Build history of the part. All positions in model axes, mm. Face numbers are marked on the shaded views. A direction names the side the tool comes from. Round coordinates to 2 decimals unless told otherwise and drop trailing zeros. Write each loop counter-clockwise with the first axis right and the second up, starting at its lowest first coordinate (ties: lowest second). Pieces come first, ordered by that corner, then holes. Notation, with made-up numbers: (53, 56) - (90, 56) arc R33 cw to (90, 86) - close; hole circle Ø8 at (70, 72.25). An arc over 180 degrees is marked (long way). Answer as a JSON object with one key per item and string values. Group by question number.
Item 1: Flat gauge pins, fed straight in: pin 1 (6.5 mm diameter, centred on x = 1, y = 3, fed in from -Z); pin 2 (1.5 mm diameter, centred on y = -2, z = 7, fed in from -X); pin 3 (1.5 mm diameter, centred on y = 5, z = 9.5, fed in from -X) (1 decimal); pin 4 (4 mm diameter, centred on x = -2.5, z = 1, fed in from +Y). Where does each tip first touch, or does it go through?
Item 2: Two-plate mould, pull along Z, no slides. Class the marked faces 1, 2 and 3: +Z half, -Z half, draft (parallel to the pull), parting line (faces both ways), or undercut.
Item 3: Which spindle directions (+Z, -Z, +X, -X, +Y, -Y) get a long thin tool onto all of the face, cutting with end or side? Do the marked faces 4, 5 and 6. Say none if no direction does.
Item 4: Slice it at D-D, the plane z = 6.75. List the corners of the cut face in (x, y), then the cut area to 3 significant figures.
Item 5: Slice it at A-A, the plane x = 0. List the corners of the cut face in (y, z).
Item 6: Slice it at B-B, the plane y = -3.25. List the corners of the cut face in (x, z), then the cut area to 3 significant figures.
Item 7: Probe line 1 (Z direction, x = 2.5, y = 0.75); line 2 (Y direction, x = -10, z = 7); line 3 (Y direction, x = 3.25, z = 15.75). List the from-to ranges inside material, lowest first. Write a range as from..to.
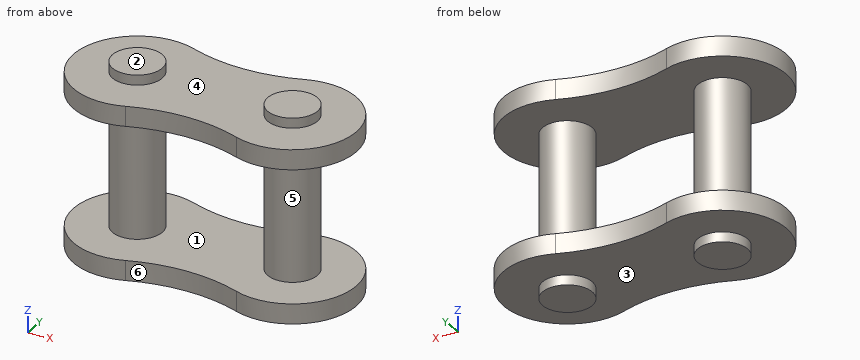
from build123d import *

# Parameters (mm, degrees)
BOSS_EXTRUDE1_DEPTH = 2.032
BOSS_EXTRUDE2_START = -3.048
SKETCH2_R           = 2.54
BOSS_EXTRUDE2_DEPTH = 16.637


# Read off the part's stored shape, not the designer's step: Boss-Extrude1
with BuildPart() as part:
    # Boss-Extrude1 outline → Boss-Extrude1 (new body)
    with BuildSketch(Plane.XY):
        with BuildLine():
            ThreePointArc((5.67954862, -6.097775113), (14.4399, 0), (5.67954862, 6.097775113))
            ThreePointArc((5.67954862, 6.097775113), (0, 5.08), (-5.67954862, 6.097775113))
            ThreePointArc((-5.67954862, 6.097775113), (-14.4399, 0), (-5.67954862, -6.097775113))
            ThreePointArc((-5.67954862, -6.097775113), (0, -5.08), (5.67954862, -6.097775113))
        make_face()
    boss_extrude1 = extrude(amount=BOSS_EXTRUDE1_DEPTH)

    # Sketch2 → Boss-Extrude2 (add)
    with BuildSketch(Plane.XY.offset(2.032).offset(BOSS_EXTRUDE2_START)):
        with Locations((-7.9375, 0)):
            Circle(SKETCH2_R)
        with Locations((7.9375, 0)):
            Circle(SKETCH2_R)
    boss_extrude2 = extrude(amount=BOSS_EXTRUDE2_DEPTH)

    # Mirror1: Boss-Extrude1, Boss-Extrude2 across plane
    add(boss_extrude1.mirror(Plane.XY.offset(8.8265)))
    add(boss_extrude2.mirror(Plane.XY.offset(8.8265)))


solid = part.part
Geometry says:
{
 "1": {"pin 1": "stops at z = 0", "pin 2": "stops at x = -10.15", "pin 3": "passes through", "pin 4": "stops at y = 5.71"},
 "2": {"face 1": "undercut", "face 2": "+Z half", "face 3": "-Z half"},
 "3": {"face 4": "+Z", "face 5": "none", "face 6": "+Z, -Z, -Y"},
 "4": {"outline": "circle Ø5.08 at (-7.94, 0); circle Ø5.08 at (7.94, 0)", "area": "40.5 mm^2"},
 "5": {"outline": "(-5.08, 0) - (5.08, 0) - (5.08, 2.03) - (-5.08, 2.03) - close; (-5.08, 15.62) - (5.08, 15.62) - (5.08, 17.65) - (-5.08, 17.65) - close"},
 "6": {"outline": "(-13.57, 0) - (13.57, 0) - (13.57, 2.03) - (-13.57, 2.03) - close; (-13.57, 15.62) - (13.57, 15.62) - (13.57, 17.65) - (-13.57, 17.65) - close", "area": "110 mm^2"},
 "7": {"line 1": "z = 0..2.03, 15.62..17.65", "line 2": "y = -1.48..1.48", "line 3": "y = -5.41..5.41"}
}
